Autodesk Inventor part; units mm, degrees
ref_plane "YZ Plane" through (0, 0, 0) normal (1, 0, 0) x (0, 1, 0)
ref_plane "XZ Plane" through (0, 0, 0) normal (0, 1, 0) x (-1, 0, 0)
ref_plane "XY Plane" through (0, 0, 0) normal (0, 0, 1) x (1, 0, 0)
sketch "Sketch1" plane through (0, 0, 0) normal (0, 0, 1) x (1, 0, 0)
  line L0 (-50, -100) -> (50, -100)
  line L1 (50, -100) -> (50, 100)
  line L2 (50, 100) -> (-50, 100)
  line L3 (-50, 100) -> (-50, -100)
  line L4 (-50, -100) -> (50, 100) construction
  line L5 (50, -100) -> (-50, 100) construction
  point P0 (0, 0)
  dimension "d0" = 100
  dimension "d1" = 200
extrude "Extrusion1" add sketch "Sketch1" along normal blind 5
sketch "Sketch2" plane through (-50, 100, 0) normal (0, 1, 0) x (1, 0, 0)
  line L0 (0, 0) -> (100, 0)
  line L1 (0, 0) -> (49.9986, 49.9986)
  line L2 (49.9986, 49.9986) -> (53.5341, 46.463)
  line L3 (53.5341, 46.463) -> (3.5355, -3.5355)
  line L4 (3.5355, -3.5355) -> (0, 0)
  line L5 (0, 0) -> (70.7086, 0) construction
  line L6 (100.108, -0.1109) -> (53.5341, 46.463)
  line L7 (53.5341, 46.463) -> (49.9986, 42.9275)
  line L8 (49.9986, 42.9275) -> (96.5724, -3.6464)
  line L9 (96.5724, -3.6464) -> (100.108, -0.1109)
  point P0 (50, 0)
  point P1 (49.9986, 42.9275)
  dimension "d4" = 45
  dimension "d5" = 5
  dimension "d6" = 5
extrude "Extrusion2" add sketch "Sketch2" against normal blind 45 contours L1 L2 L3 L0 | L0 L3 L4 | L8 L3 L6 L0 | L0 L6 L9 L8
sketch "Sketch6" plane through (0, 0, 5) normal (0, 0, 1) x (1, 0, 0)
  line L0 (4.9986, 75) -> (-5.0014, 75)
  line L1 (-25.0014, 55) -> (-25.0014, 45)
  line L2 (-5.0014, 25) -> (4.9986, 25)
  line L3 (24.9986, 45) -> (24.9986, 55)
  line L4 (24.9986, 75) -> (-25.0014, 25) construction
  line L5 (-25.0014, 75) -> (24.9986, 25) construction
  arc A0 (4.9986, 25) -> (24.9986, 45) centre (4.9986, 45) ccw
  arc A1 (24.9986, 55) -> (4.9986, 75) centre (4.9986, 55) ccw
  arc A2 (-5.0014, 75) -> (-25.0014, 55) centre (-5.0014, 55) ccw
  arc A3 (-25.0014, 45) -> (-5.0014, 25) centre (-5.0014, 45) ccw
  point P0 (0, 0)
  point P1 (-0.0014, 50)
  dimension "d21" = 50
  dimension "d22" = 50
  dimension "d23" = 20
extrude "Extrusion6" cut sketch "Sketch6" against normal blind 5
sketch "Sketch10" plane through (-50, 100, 5) normal (0, 1, 0) x (1, 0, 0)
  line L0 (0, 5) -> (7.0711, 5)
  line L1 (49.9986, 54.9986) -> (99.9971, 5)
  line L2 (0, 5) -> (49.9986, 54.9986)
  line L3 (49.9986, 54.9986) -> (46.463, 58.5341)
  line L4 (46.463, 58.5341) -> (-3.5355, 8.5355)
  line L5 (-3.5355, 8.5355) -> (0, 5)
  line L6 (100, 4.7812) -> (100, 0)
  line L7 (100, 4.7812) -> (49.9986, 54.9986)
  line L8 (49.9986, 54.9986) -> (53.5417, 58.5265)
  line L9 (53.5417, 58.5265) -> (103.5431, 8.3091)
  line L10 (103.5431, 8.3091) -> (100, 4.7812)
  line L11 (92.926, 5) -> (49.9986, 47.9275)
  line L12 (100, 0) -> (0, 0)
  line L13 (0, 0) -> (100, 0)
  point P0 (50, 5)
  dimension "d33" = 5
  dimension "d34" = 5
extrude "Extrusion9" add sketch "Sketch10" against normal blind 3
properties part number "fixation_v07"
Here's how the part is built. I have some questions about the finished solid (model axes, mm). A direction names the side the tool comes from. Coordinates: 2 decimals unless noted, no trailing zeros. Loops run counter-clockwise (first coordinate to the right, second up) from the corner with the lowest first, then second, coordinate; pieces in that order, holes last. Notation, with made-up numbers: (65.5, 49.25) -> (96.5, 49.25) arc R18 cw to (96.5, 78.25) -> close; hole circle Ø10 at (62.25, 12.25). An arc over 180 degrees is marked (long way). Use one line per item in the form item = value. Start each with the question number.
(1) We'd pull the mould along Y, two halves only. Please class faces 4 (the face through (8.2, 100, -35.2)), 5 (the face through (-11, 55, -33)), 6 (the face through (19.295, 68.986, 2.535)): pulls with the +Y half, pulls with the -Y half, needs draft (parallel to the pull), parting line crosses it, or undercut.
(2) If we section it at C-C (z = -41): Please give me the cut outline in (x, y).
(3) Please list where these lines run through material, in increasing order: line 1 along X through (y, z) = (76, 2.5); line 2 along Z through (x, y) = (-6.5, -68.5); line 3 along Z through (x, y) = (-42.5, 83).
(4) If we section it at B-B (x = 39.5): Please give me the cut outline in (y, z), then the cut area to 3 significant figures.
(5) If we section it at D-D (x = -22): Please give me the cut outline in (y, z).
(6) If we section it at A-A (x = -8.5): Please give me the cut outline in (y, z), then the cut area to 3 significant figures.
(7) On a 3-axis mill with a long thin cutter (end or side, diameter ignored), from which of +Z, -Z, +X, -X, +Y, -Y can I reach the whole of each face in a straight line? I mean faces 1 (the face through (-25, 76, -25)), 2 (the face through (-21.165, 77.815, -21.764)), 3 (the face through (24.999, 50, 3)). Say none if no direction works.
(8) Will these pins go through, and if not, where does the flat tip stop? pin 1 (25 mm diameter, centred on x = -8.5, z = -21, fed in from -Y); pin 2 (1.5 mm diameter, centred on y = 52, z = 2, fed in from -X); pin 3 (10 mm diameter, centred on x = -7.5, z = -26, fed in from -Y); pin 4 (1.5 mm diameter, centred on y = 74.5, z = -35, fed in from -X).
Verdict:
q1.face_4 = pulls with the +Y half
q1.face_5 = pulls with the -Y half
q1.face_6 = undercut
q2.outline = (-16.07, 97) -> (-9, 97) -> (-9, 55) -> (-1.93, 55) -> (-1.93, 100) -> (-16.07, 100) -> close; (1.93, 55) -> (9, 55) -> (9, 97) -> (16.01, 97) -> (16.01, 100) -> (1.93, 100) -> close
q3.line_1 = -50 to 50
q3.line_2 = 0 to 5
q3.line_3 = -7.5 to -0.43, 0 to 5
q4.outline = (-100, 0) -> (100, 0) -> (100, 5) -> (-100, 5) -> close; (55, -10.5) -> (97, -10.5) -> (97, -17.41) -> (100, -17.41) -> (100, -3.43) -> (55, -3.43) -> close
q4.area = 1,340 mm²
q5.outline = (-100, 0) -> (34.46, 0) -> (34.46, 5) -> (-100, 5) -> close; (55, -28) -> (97, -28) -> (97, -35.07) -> (100, -35.07) -> (100, -20.93) -> (55, -20.93) -> close; (65.54, 0) -> (100, 0) -> (100, 5) -> (65.54, 5) -> close
q6.outline = (-100, 0) -> (25.31, 0) -> (25.31, 5) -> (-100, 5) -> close; (55, -41.5) -> (97, -41.5) -> (97, -48.57) -> (100, -48.57) -> (100, -34.43) -> (55, -34.43) -> close; (74.69, 0) -> (100, 0) -> (100, 5) -> (74.69, 5) -> close
q6.area = 1,090 mm²
q7.face_1 = -Z, -X, -Y
q7.face_2 = +Y, -Y
q7.face_3 = +Z, -Z
q8.pin_1 = 55
q8.pin_2 = -50
q8.pin_3 = through
q8.pin_4 = -15.75
